from build123d import *

# Parameters (mm, degrees)
PAD001_DEPTH    = 5
SKETCH009_R     = 35
SKETCH009_R_2   = 1.6
POCKET002_DEPTH = 5.001
SKETCH010_R     = 3.5
SKETCH010_R_2   = 1.7
POCKET003_DEPTH = 5.001
COPYSKETCH026_W = 39
COPYSKETCH026_H = 51
POCKET029_DEPTH = 7.5
SKETCH034_W     = 8
SKETCH034_H     = 15
POCKET035_DEPTH = 5.001


with BuildPart() as part:
    # Sketch008 → Pad001 (new body)
    with BuildSketch(Plane.XY):
        with BuildLine():
            Line((0, 67.42), (0, -55.65))
            Line((0, -55.65), (-117.94, -55.65))
            ThreePointArc((-127.64, -49.11), (-122.947197, -52.613151), (-117.94, -55.65))
            ThreePointArc((-146.95, -26.77), (-138.520798, -38.999541), (-127.64, -49.11))
            ThreePointArc((-148.54, 6.09), (-150.980867, -10.496574), (-146.95, -26.77))
            ThreePointArc((-134.5, 26.2), (-142.831473, 17.060618), (-148.54, 6.09))
            ThreePointArc((-94.13, 48.54), (-115.023795, 38.650843), (-134.5, 26.2))
            ThreePointArc((0, 67.42), (-48.036997, 62.826084), (-94.13, 48.54))
        make_face()
    extrude(amount=PAD001_DEPTH)

    # Sketch009 (on Face10 of Pad001) → Pocket002 (cut, through all)
    with BuildSketch(Plane.XY.offset(5)):
        with Locations((-90.05, -4.36)):
            Circle(SKETCH009_R)
        with Locations((-119.571708, 25.161708)):
            Circle(SKETCH009_R_2)
        with Locations((-119.571708, -33.881708)):
            Circle(SKETCH009_R_2)
        with Locations((-60.528292, -33.881708)):
            Circle(SKETCH009_R_2)
        with Locations((-60.528292, 25.161708)):
            Circle(SKETCH009_R_2)
    extrude(amount=-POCKET002_DEPTH, mode=Mode.SUBTRACT)

    # Sketch010 (on Face5 of Pocket002) → Pocket003 (cut, through all)
    with BuildSketch(Plane.XY.offset(5)):
        with Locations((-30, -40)):
            Circle(SKETCH010_R)
        with Locations((-35.05, 21.8)):
            Circle(SKETCH010_R_2)
        with Locations((-35.05, -21.8)):
            Circle(SKETCH010_R_2)
        Polygon((0, 25.5), (-30.35, 25.5), (-30.35, 18.5), (-38.25, 18.5), (-38.25, -18.5), (-30.35, -18.5), (-30.35, -25.5), (0, -25.5), align=None)
    extrude(amount=-POCKET003_DEPTH, mode=Mode.SUBTRACT)

    # CopySketch026 → Pocket029 (cut)
    with BuildSketch(Plane.XY.offset(10)):
        with Locations((-19.5, 0)):
            Rectangle(COPYSKETCH026_W, COPYSKETCH026_H)
    extrude(amount=-POCKET029_DEPTH, mode=Mode.SUBTRACT)

    # Sketch034 (on Face5 of Pocket029) → Pocket035 (cut, through all)
    with BuildSketch(Plane.XY.offset(5)):
        with Locations((-42, 0)):
            Rectangle(SKETCH034_W, SKETCH034_H)
    extrude(amount=-POCKET035_DEPTH, mode=Mode.SUBTRACT)


with BuildPart() as part_1:
    # Body001 placement: moved
    add(part.part.moved(Location((0, 0, -3))))


solid = part_1.part
Read the model definition and answer for the solid it produces. Units are mm, in the model's axes. A direction names the side the tool comes from. Coordinates: 2 decimals unless noted, no trailing zeros. Order: outer loops, then holes, each group sorted by start corner. A loop starts at its lowest first (then second) coordinate and runs counter-clockwise, first axis right, second up. Notation, with made-up numbers: M 19.25,-18 L 58.25,-18 A15 ccw 58.25,5 Z; hole C 76,64.5 d6. An arc over 180 degrees is marked long. Put each result on its own line as item: value. Start each with the question number.
Item 1: Section A-A, the plane y = -12 is taken. Determine the outline of the cut face in (x, z).
Item 2: Section B-B, the plane x = -90.05 is taken. Determine the outline of the cut face in (y, z), plus the area to 3 significant figures.
Item 3: Section C-C, the plane y = 21.8 is taken. Determine the outline of the cut face in (x, z), plus the area to 3 significant figures.
Item 4: Given pin 1 Ø2 at (y, z) = (-22, -2) entering from +X; pin 2 Ø1.5 at (y, z) = (1, -1.5) entering from +X; pin 3 Ø7 at (x, y) = (-32.5, 13) entering from +Z; pin 4 Ø1.2 at (y, z) = (-17, 0.5) entering from +X, each flat-ended and moving along its own axis, determine where each tip first touches the part or whether it passes through.
Item 5: The mould has two halves that part along X. Classify faces 1 (the face through (-142.732, 17.203, -0.535)), 2 (the face through (-58, 20, 2)), 3 (the face through (-59.05, 24.55, -0.46)): +X half, -X half, draft (parallel to the pull), parting line (faces both ways), or undercut.
Item 6: Consider probe 1 along Y at (x, z) = (-35.05, -1.8); probe 2 along X at (y, z) = (-29, -0.8); probe 3 along Y at (x, z) = (-9.5, -1.9). Determine where each line is inside the solid, lowest interval first. Write a range as [from, to].
Item 7: Section D-D, the plane z = 1.2 is taken. Determine the outline of the cut face in (x, y).
Item 8: For faces 4 (the face through (-42, 7.5, 0)), 5 (the face through (-114.74, 38.807, -0.535)), 6 (the face through (-37, 21, -0.5)), determine the directions among +Z, -Z, +X, -X, +Y, -Y from which every point of the face is accessible in a straight line to the end or side of a thin tool.
Computed:
1. outline: M -150.88,-3 L -124.21,-3 L -124.21,2 L -150.88,2 Z; M -55.89,-3 L -38.25,-3 L -38.25,-0.5 L -39,-0.5 L -39,2 L -55.89,2 Z
2. outline: M -55.65,-3 L -39.36,-3 L -39.36,2 L -55.65,2 Z; M 30.64,-3 L 50.24,-3 L 50.24,2 L 30.64,2 Z
2. area: 179 mm2
3. outline: M -139.05,-3 L -113.3,-3 L -113.3,2 L -139.05,2 Z; M -66.8,-3 L -36.75,-3 L -36.75,-0.5 L -39,-0.5 L -39,2 L -66.8,2 Z; M -33.35,-3 L -30.35,-3 L -30.35,-0.5 L -33.35,-0.5 Z
3. area: 281 mm2
4. pin 1: stops at x = -30.35
4. pin 2: stops at x = -46
4. pin 3: passes through
4. pin 4: stops at x = -39
5. face 1: -X half
5. face 2: draft
5. face 3: undercut
6. probe 1: y = [-55.65, -23.5], [-20.1, -18.5], [18.5, 20.1], [23.5, 65.06]
6. probe 2: x = [-145.69, -114.91], [-65.19, 0]
6. probe 3: y = [-55.65, -25.5], [25.5, 67.3]
7. outline: M -148.54,6.09 A43.38 ccw -146.95,-26.77 A68.08 ccw -127.64,-49.11 A60.98 ccw -117.94,-55.65 L 0,-55.65 L 0,-25.5 L -39,-25.5 L -39,-7.5 L -46,-7.5 L -46,7.5 L -39,7.5 L -39,25.5 L 0,25.5 L 0,67.42 A235.57 ccw -94.13,48.54 A182.51 ccw -134.5,26.2 A47.81 ccw Z; hole C -90.05,-4.36 d70; hole C -119.57,-33.88 d3.2; hole C -119.57,25.16 d3.2; hole C -60.53,-33.88 d3.2; hole C -60.53,25.16 d3.2; hole C -30,-40 d7
8. face 4: +Z, -Z, +X
8. face 5: +Z, -Z, -X, +Y
8. face 6: +Z, +X
